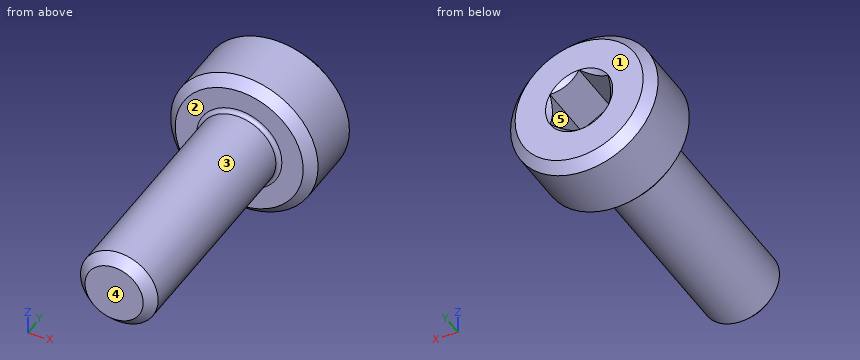
Autodesk Inventor part; units mm, degrees
ref_plane "YZ Plane" through (0, 0, 0) normal (1, 0, 0) x (0, 1, 0)
ref_plane "XZ Plane" through (0, 0, 0) normal (0, 1, 0) x (-1, 0, 0)
ref_plane "XY Plane" through (0, 0, 0) normal (0, 0, 1) x (1, 0, 0)
sketch "Sketch1" plane through (0, 0, 0) normal (0, 0, 1) x (1, 0, 0)
  line L0 (0, 4) -> (0, -4)
  line L1 (0, -4) -> (0.75, -4)
  line L2 (0.75, -4) -> (1, -3.75)
  line L3 (1, -3.75) -> (1, 1.9)
  line L4 (1.1, 2) -> (1.65, 2)
  line L5 (1.9, 2.25) -> (1.9, 3.75)
  line L6 (1.65, 4) -> (0, 4)
  arc A0 (1.1, 2) -> (1, 1.9) centre (1.1, 1.9) ccw
  line L7 (1.65, 4) -> (1.9, 3.75)
  line L8 (1.65, 2) -> (1.9, 2.25)
  point P0 (0, 0)
  point P1 (1.9, 2)
  point P2 (1.9, 4)
  point P3 (0, 0)
  dimension "d0" = 3.8
  dimension "d1" = 2
  dimension "d3" = 2
  dimension "d4" = 2.2
  dimension "d5" = 135
  dimension "d6" = 0.25
  dimension "d7" = 6
  dimension "d18" = 0.25
revolve "Revolution1" add sketch "Sketch1" angle 360 about axis through (0, 4, 0) along (0, -1, 0)
sketch "Sketch2" plane through (0, 4, 0) normal (0, 1, 0) x (1, 0, 0)
  line L0 (0, -0.866) -> (-0.75, -0.433)
  line L1 (-0.75, -0.433) -> (-0.75, 0.433)
  line L2 (-0.75, 0.433) -> (0, 0.866)
  line L3 (0, 0.866) -> (0.75, 0.433)
  line L4 (0.75, 0.433) -> (0.75, -0.433)
  line L5 (0.75, -0.433) -> (0, -0.866)
  point P0 (0, 0)
  point P1 (0, 0)
  dimension "d11" = 1.5
extrude "Extrusion1" cut sketch "Sketch2" against normal blind 1.5
thread "Thread1"
sketch "Sketch3" plane through (0, 0, 0) normal (1, 0, 0) x (0, 1, 0)
  line L0 (4, 0.866) -> (4, 0.433)
  line L1 (4, 0.866) -> (3.5, 0.366)
  line L2 (3.5, 0.366) -> (4, 0.366)
  line L3 (4, 0.366) -> (4, 0.866)
  line L4 (-0.8, 0) -> (4.8, 0)
  point P0 (0, 0)
  dimension "d16" = 0.5
revolve "Revolution2" cut sketch "Sketch3" angle 360 about axis through (0, -10, 0) along (0, 1, 0)
properties part number "Bolt_M2x0.4_6mm_SH" material "Stainless Steel"
Can you work these out from the model? Positions are in its coordinate system, mm. Face numbers are marked on the shaded views. A direction names the side the tool comes from. Round coordinates to 2 decimals unless told otherwise and drop trailing zeros. Order: outer loops, then holes, each group sorted by start corner. A loop starts at its lowest first (then second) coordinate and runs counter-clockwise, first axis right, second up. Notation, with made-up numbers: M -35.75,38 L -26.75,38 A16 ccw -26.75,68 Z; hole C -31.5,54 d1. An arc over 180 degrees is marked long. Use a Markdown table: item, result.
1) On a 3-axis mill with a long thin cutter (end or side, diameter ignored), from which of +Z, -Z, +X, -X, +Y, -Y can I reach the whole of each face in a straight line? I mean the marked faces 1 and 2. Say none if no direction works.
Geometry says:
| item | result |
|---|---|
| face 1 | +Z, -Z, +X, -X, +Y |
| face 2 | -Y |
2) Imagine slicing it at A-A (z = 0). List the corners of the cut face in (x, y) for me.
Geometry says:
| item | result |
|---|---|
| outline | M -1.9,2.25 L -1.65,2 L -1.1,2 A0.1 cw -1,1.9 L -1,-3.75 L -0.75,-4 L 0.75,-4 L 1,-3.75 L 1,1.9 A0.1 cw 1.1,2 L 1.65,2 L 1.9,2.25 L 1.9,3.75 L 1.65,4 L 0.87,4 L 0.75,3.88 L 0.75,2.5 L -0.75,2.5 L -0.75,3.88 L -0.87,4 L -1.65,4 L -1.9,3.75 Z |
3) I'm going to push flat-ended pins straight in: P1, Ø2, axis at x = -1.5, z = 1, coming from the +Y side; P2, Ø1, axis at x = -1.5, z = 1.5, coming from the -Y side. Where does each tip first touch, or does it pass through?
Geometry says:
| item | result |
|---|---|
| P1 | stops at y = 4 |
| P2 | stops at y = 2 |
4) If I drill on line 1 along Y through (x, z) = (0.4, 1.5); line 2 along Z through (x, y) = (-0.6, 3); line 3 along Z through (x, y) = (-0.5, -0.5), over which ranges is the centre line in solid material (lowest first)?
Geometry says:
| item | result |
|---|---|
| line 1 | y = 2 to 4 |
| line 2 | z = -1.8 to -0.52, 0.52 to 1.8 |
| line 3 | z = -0.87 to 0.87 |
5) If we mould it in two halves opening along X, with no side actions, what happens to the marked faces 3, 4 and 5? For each: +X half, -X half, draft (parallel to the pull), parting line (faces both ways), or undercut.
Geometry says:
| item | result |
|---|---|
| face 3 | parting line |
| face 4 | draft |
| face 5 | undercut |
6) Imagine slicing it at B-B (y = 1.5). List the corners of the cut face in (x, z) for me.
Geometry says:
| item | result |
|---|---|
| outline | C 0,0 d2 |
